```python
from build123d import *

# Parameters (mm, degrees)
SKETCH1_W           = 125
SKETCH1_H           = 70
SKETCH1_R           = 1.6
SKETCH1_R_2         = 1.5
BOSS_EXTRUDE1_DEPTH = 5
FILLET1_R           = 2


with BuildPart() as part:
    # Sketch1 → Boss-Extrude1 (new body)
    with BuildSketch(Plane.XY):
        with Locations((62.5, 35)):
            Rectangle(SKETCH1_W, SKETCH1_H)
        with Locations((15, 55)):
            Circle(SKETCH1_R, mode=Mode.SUBTRACT)
        with Locations((13.73, 6.8)):
            Circle(SKETCH1_R, mode=Mode.SUBTRACT)
        with Locations((82.573533757, 6.8)):
            Circle(SKETCH1_R, mode=Mode.SUBTRACT)
        with Locations((89.9, 55)):
            Circle(SKETCH1_R, mode=Mode.SUBTRACT)
        with Locations((65.8, 39.8)):
            Circle(SKETCH1_R, mode=Mode.SUBTRACT)
        with Locations((65.8, 11.9)):
            Circle(SKETCH1_R, mode=Mode.SUBTRACT)
        with Locations((2.5, 67.5)):
            Circle(SKETCH1_R_2, mode=Mode.SUBTRACT)
        with Locations((122.5, 67.5)):
            Circle(SKETCH1_R_2, mode=Mode.SUBTRACT)
        with Locations((122.5, 2.5)):
            Circle(SKETCH1_R_2, mode=Mode.SUBTRACT)
        with Locations((2.5, 2.5)):
            Circle(SKETCH1_R_2, mode=Mode.SUBTRACT)
    extrude(amount=BOSS_EXTRUDE1_DEPTH)

    # Fillet1
    fillet1_edges = [part.edges().sort_by_distance(p)[0] for p in [
        (0, 70, 2.5),
        (125, 70, 2.5),
        (125, 0, 2.5),
        (0, 0, 2.5),
    ]]
    fillet(fillet1_edges, radius=FILLET1_R)


solid = part.part
```
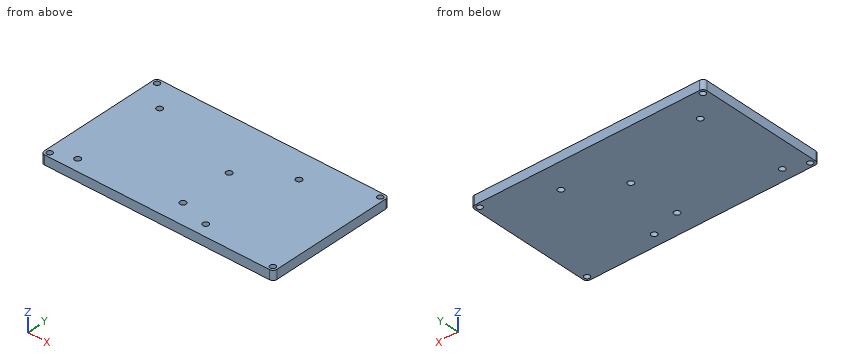
The listing builds one solid part. Answer for the finished solid, in the listing's coordinates (mm). Round coordinates to 2 decimals unless told otherwise and drop trailing zeros. Write each loop counter-clockwise with the first axis right and the second up, starting at its lowest first coordinate (ties: lowest second). Pieces come first, ordered by that corner, then holes. Notation, with made-up numbers: (70.25, 44) -> (83.25, 44) arc R10 ccw to (83.25, 60) -> close; hole circle Ø8 at (83.25, 2.25). An arc over 180 degrees is marked (long way). Answer as a JSON object with one key per item and string values. Group by question number.
Q1. Section C-C (y = 6.8) is taken. Write down the section's boundary in (x, z).
Q2. Section B-B (x = 89.9) is taken. Write down the section's boundary in (y, z), plus the area to 3 significant figures.
Q3. This flat-tipped pin is pushed along its axis until it touches: pin 1 Ø2.5 at (x, y) = (122.5, 2.5) entering from -Z. Where does it stop, or does it pass through?
Q4. Straight lines are drawn through the part: line 1 along Y through (x, z) = (122.5, 2.45); line 2 along Y through (x, z) = (65.8, 3.3); line 3 along X through (y, z) = (56, 2.4). For each, find the intervals that lie inside material, in ascending order.
Q5. Section A-A (y = 39.8) is taken. Write down the section's boundary in (x, z), plus the area to 3 significant figures.
Check values:
{
 "1": {"outline": "(0, 0) -> (12.13, 0) -> (12.13, 5) -> (0, 5) -> close; (15.33, 0) -> (80.97, 0) -> (80.97, 5) -> (15.33, 5) -> close; (84.17, 0) -> (125, 0) -> (125, 5) -> (84.17, 5) -> close"},
 "2": {"outline": "(0, 0) -> (53.4, 0) -> (53.4, 5) -> (0, 5) -> close; (56.6, 0) -> (70, 0) -> (70, 5) -> (56.6, 5) -> close", "area": "334 mm^2"},
 "3": {"pin 1": "through"},
 "4": {"line 1": "0 to 1, 4 to 66, 69 to 70", "line 2": "0 to 10.3, 13.5 to 38.2, 41.4 to 70", "line 3": "0 to 13.75, 16.25 to 88.65, 91.15 to 125"},
 "5": {"outline": "(0, 0) -> (64.2, 0) -> (64.2, 5) -> (0, 5) -> close; (67.4, 0) -> (125, 0) -> (125, 5) -> (67.4, 5) -> close", "area": "609 mm^2"}
}
